Source: CAD feature listing. Evaluate the final solid. Frame: model axes, mm. Face numbers are marked on the shaded views. Give positions to 0.01 mm unless a question says otherwise; leave off trailing zeros. Write each loop counter-clockwise with the first axis right and the second up, starting at its lowest first coordinate (ties: lowest second). Pieces come first, ordered by that corner, then holes. Notation, with made-up numbers: (31.5, 40) -> (70.5, 40) arc R18 ccw to (70.5, 67) -> close; hole circle Ø3 at (-29.5, -29.5). An arc over 180 degrees is marked (long way). Use one line per item in the form item = value. Start each with the question number.
(1) Cut plane A-A, the plane y = 3.45. Output: boundary loops of the cut face in (x, z).
(2) Cut plane B-B, the plane y = 4.1. Output: boundary loops of the cut face in (x, z), and give its area (3 significant figures).
(3) Draft query along Z for the marked faces 1, 2, 3 and 4. Return one class per face: pulls with the +Z half, pulls with the -Z half, needs draft (parallel to the pull), parting line crosses it, or undercut.
(4) Material intervals for line 1 along X through (y, z) = (2.5, 0.5); line 2 along Z through (x, y) = (-0.5, 3.1); line 3 along X through (y, z) = (3.2, -0.25), sorted ascending. Write a range as from..to.
from build123d import *

# Parameters (mm, degrees)
SKETCH1_R           = 2
BOSS_EXTRUDE1_DEPTH = 5
SKETCH2_OUTSIDE_W   = 25.558
SKETCH2_OUTSIDE_H   = 24.218
SKETCH2_OUTSIDE_R   = 4.330127019
CUT_EXTRUDE1_DEPTH  = 9.291561976
CUT_EXTRUDE1_DRAFT  = -30


with BuildPart() as part:
    # Sketch1 → Boss-Extrude1 (new body)
    with BuildSketch(Plane(origin=(0, 0, 0), x_dir=(1, 0, 0), z_dir=(0, 1, 0))):
        Polygon((5, 0), (2.5, 4.330127019), (-2.5, 4.330127019), (-5, 0), (-2.5, -4.330127019), (2.5, -4.330127019), align=None)
        with Locations(Location((0, 0, 0), (0, 0, 270))):
            Circle(SKETCH1_R, mode=Mode.SUBTRACT)
    extrude(amount=BOSS_EXTRUDE1_DEPTH)


with BuildPart() as cut_extrude1_tool:
    # Sketch2 outside → Cut-Extrude1 (with draft: the straight prism first)
    with BuildSketch(Plane(origin=(0, 5, 0), x_dir=(1, 0, 0), z_dir=(0, 1, 0))):
        Rectangle(SKETCH2_OUTSIDE_W, SKETCH2_OUTSIDE_H)
        Circle(SKETCH2_OUTSIDE_R, mode=Mode.SUBTRACT)
    extrude(amount=-CUT_EXTRUDE1_DEPTH)
    # Cut-Extrude1: the draft: its side faces are tilted about the plane it starts from
    cut_extrude1_sides = [cut_extrude1_tool.faces().sort_by_distance(p)[0] for p in [
        (0, 0.354219012, 12.109),
        (12.779, 0.354219012, 0),
        (0, 0.354219012, -12.109),
        (-12.779, 0.354219012, 0),
        (-4.330127019, 0.354219012, 0),
    ]]
    draft(cut_extrude1_sides, Plane(origin=(0, 5, 0), x_dir=(1, 0, 0), z_dir=(0, 1, 0)), CUT_EXTRUDE1_DRAFT)


with BuildPart() as part_1:
    add(part.part)

    # Cut-Extrude1: cut by cut_extrude1_tool
    add(cut_extrude1_tool.part, mode=Mode.SUBTRACT)


solid = part_1.part
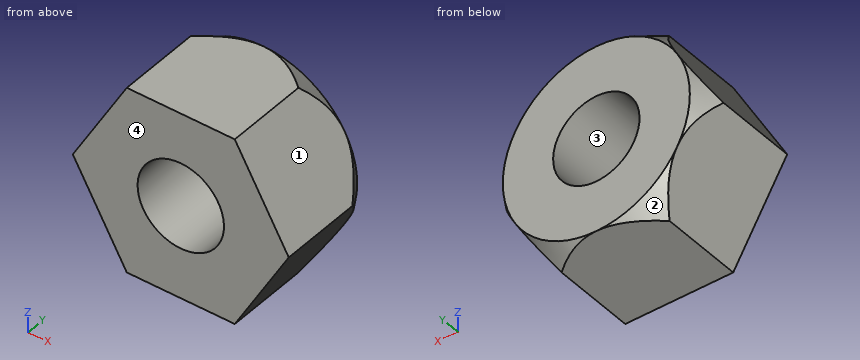
Geometry says:
q1.outline = (-5, 0) -> (-2.5, -4.33) -> (2.5, -4.33) -> (5, 0) -> (2.5, 4.33) -> (-2.5, 4.33) -> close; hole circle Ø4 at (0, 0)
q2.outline = (-4.84, -0.27) -> (-2.66, -4.06) arc R4.85 ccw to (-2.18, -4.33) -> (2.18, -4.33) arc R4.85 ccw to (2.66, -4.06) -> (4.84, -0.27) arc R4.85 ccw to (4.84, 0.27) -> (2.66, 4.06) arc R4.85 ccw to (2.18, 4.33) -> (-2.18, 4.33) arc R4.85 ccw to (-2.66, 4.06) -> (-4.84, 0.27) arc R4.85 ccw to start; hole circle Ø4 at (0, 0)
q2.area = 52.1 mm^2
q3.face_1 = pulls with the +Z half
q3.face_2 = pulls with the -Z half
q3.face_3 = undercut
q3.face_4 = needs draft
q4.line_1 = -4.71..-1.94, 1.94..4.71
q4.line_2 = -4.33..-1.94, 1.94..4.33
q4.line_3 = -4.86..-1.98, 1.98..4.86
